Answer from the drawing. Dimensions are ordinates in mm from the lowest x, y and z of the part. Coordinates: 2 decimals unless noted, no trailing zeros. Write each loop counter-clockwise with the first axis right and the second up, starting at its lowest first coordinate (ties: lowest second). Pieces come first, ordered by that corner, then holes. Notation, with made-up numbers: (75.5, 59.25) -> (115.5, 59.25) arc R18 cw to (115.5, 86.25) -> close; hole circle Ø4 at (-35.5, -24.75). An arc over 180 degrees is marked (long way). Answer as a JSON object with one key per item and string values. Group by question number.
(1) Flat-ended cylindrical pins translate along their axes: P1, Ø5, axis at x = 244.5, y = 195, coming from the +Z side (1 decimal); P2, Ø1.4, axis at x = 244.5, z = 6.5, coming from the +Y side; P3, Ø1.4, axis at x = 245, z = 7, coming from the -Y side (1 decimal). Find the tip coordinate at first contact, or state that the pin passes through.
(2) Find section B-B (z = 22). Give the vertices of the cut face in (x, y) (1 decimal), then the cut area to 3 significant figures.
(3) Find section D-D (y = 122). Give the vertices of the cut face in (x, z).
(4) Straight lines are drawn through the part: L1, parallel to X at y = 213.5, z = 10; L2, parallel to X at y = 41.5, z = 7.5. For each, find the intervals that lie inside material, in ascending order.
(5) Find section C-C (x = 140.5). Give the vertices of the cut face in (y, z) (1 decimal).
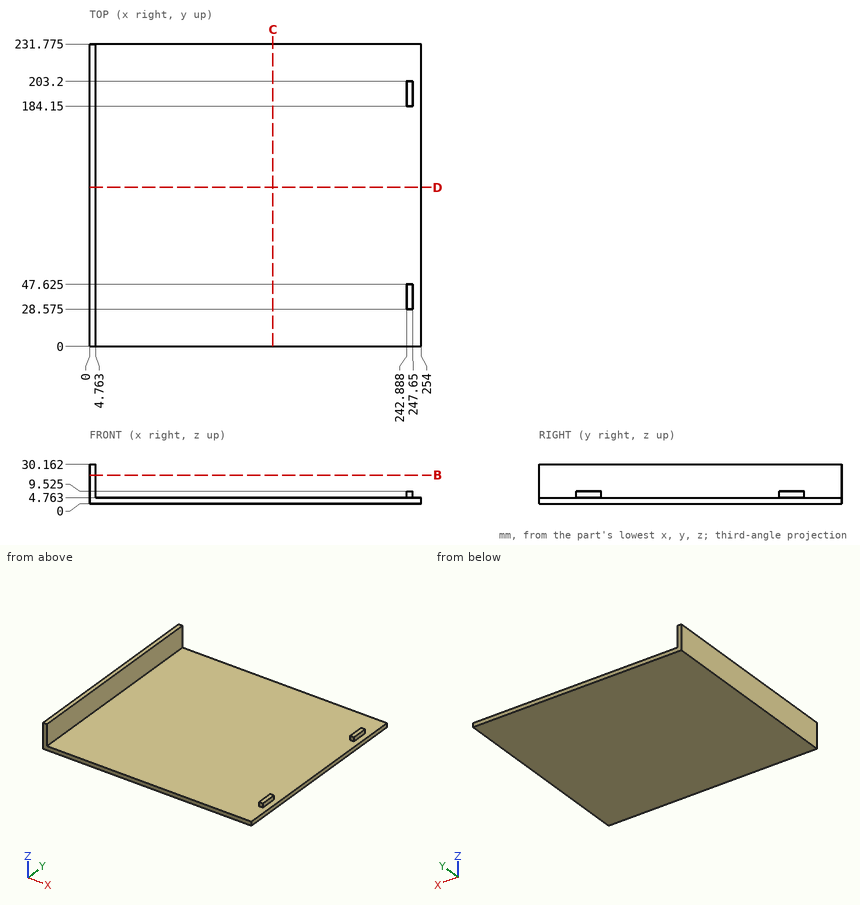
Results below:
{
 "1": {"P1": "stops at z = 9.5", "P2": "stops at y = 203.2", "P3": "stops at y = 28.6"},
 "2": {"outline": "(0, 0) -> (4.8, 0) -> (4.8, 231.8) -> (0, 231.8) -> close", "area": "1,100 mm2"},
 "3": {"outline": "(0, 0) -> (254, 0) -> (254, 4.76) -> (4.76, 4.76) -> (4.76, 30.16) -> (0, 30.16) -> close"},
 "4": {"L1": "x = 0 to 4.76", "L2": "x = 0 to 4.76, 242.89 to 247.65"},
 "5": {"outline": "(0, 0) -> (231.8, 0) -> (231.8, 4.8) -> (0, 4.8) -> close"}
}
